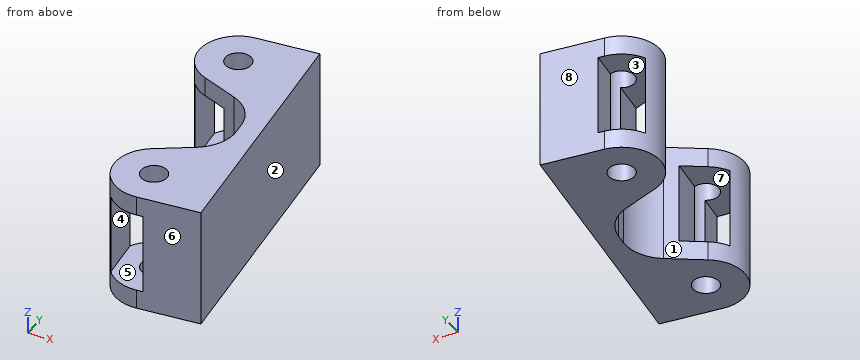
from build123d import *

# Parameters (mm, degrees)
SKETCH2_R           = 4
BOSS_EXTRUDE1_DEPTH = 18.5
SKETCH3_W           = 11.7897503
SKETCH3_H           = 96.005071975
CUT_EXTRUDE1_DEPTH  = 12.5


with BuildPart() as part:
    # Sketch2 → Boss-Extrude1 (new body, symmetric)
    with BuildSketch(Plane(origin=(137.548518754, -674.152855032, 0), x_dir=(0.993680552, 0.112245088, 0), z_dir=(0, 0, -1))):
        with BuildLine():
            Line((9.525, -304.744352791), (28.575, -304.744352791))
            Line((28.575, -304.744352791), (28.575, -387.05564726))
            Line((28.575, -387.05564726), (9.525993953, -387.05564726))
            ThreePointArc((9.525993953, -387.05564726), (-2.161189853, -377.777730047), (4.223746974, -364.290603044))
            Line((4.223746974, -364.290603044), (15.13654472, -358.9155811))
            ThreePointArc((15.13654472, -358.9155811), (20.308242044, -354.231651246), (22.225, -347.522575972))
            Line((22.225, -347.522575972), (22.225, -344.276661697))
            ThreePointArc((22.225, -344.276661697), (20.30793231, -337.567088625), (15.135492786, -332.883138506))
            Line((15.135492786, -332.883138506), (4.223746974, -327.509886515))
            ThreePointArc((4.223746974, -327.509886515), (-2.162309457, -314.022809542), (9.525, -304.744352791))
        make_face()
        with Locations((9.525993953, -375.05564726)):
            Circle(SKETCH2_R, mode=Mode.SUBTRACT)
        with Locations((9.525, -316.744352791)):
            Circle(SKETCH2_R, mode=Mode.SUBTRACT)
    extrude(amount=BOSS_EXTRUDE1_DEPTH, both=True)

    # Sketch3 → Cut-Extrude1 (cut, symmetric)
    with BuildSketch(Plane(origin=(140.134572942, -673.053475883, 0), x_dir=(0.993680552, 0.112245088, 0), z_dir=(0, 0, -1))):
        with Locations((2.760437102, -344.382335899)):
            Rectangle(SKETCH3_W, SKETCH3_H)
    extrude(amount=CUT_EXTRUDE1_DEPTH, both=True, mode=Mode.SUBTRACT)


solid = part.part
Geometry check sheet. Reference: the model listing, model coordinates, mm. Face numbers are marked on the shaded views. A direction names the side the tool comes from. Give positions to 0.01 mm unless a question says otherwise; leave off trailing zeros. Write each loop counter-clockwise with the first axis right and the second up, starting at its lowest first coordinate (ties: lowest second). Pieces come first, ordered by that corner, then holes.
1) Thickness scan on line 1 (Z direction, x = 111, y = -348.5); line 2 (Y direction, x = 113.5, z = 15); line 3 (X direction, y = -299.5, z = -11). Record the ranges inside material, lowest first.
Values follow:
line 1: z = -18.5 to -12.5, 12.5 to 18.5
line 2: y = -370.19 to -361.78, -354.9 to -342.78, -316.31 to -287.35
line 3: x = 92.95 to 94.78, 108.81 to 123.98
2) Release check for a two-part mould opening along X. For the marked faces 5, 6, 7 and 8 record: released by +X, released by -X, zero draft, split by the parting line, or undercut.
Values follow:
face 5: undercut
face 6: released by +X
face 7: undercut
face 8: released by -X
3) Cross-section at A-A (z = -3). Record the boundary of the cut face in (x, y), plus the area to 3 significant figures.
Values follow:
outline: (94.26, -294.88) arc R12 ccw to (95.76, -308.16) - close; (100.81, -352.82) arc R12 ccw to (102.31, -366.1) - close; (105.38, -288.27) - (106.33, -296.66) arc R4 cw to (107.13, -303.73) - (108.33, -314.38) - (112.3, -315.81) arc R12.7 cw to (120.63, -326.33) - (120.99, -329.56) arc R12.7 cw to (115.22, -341.67) - (111.67, -343.95) - (112.87, -354.6) arc R4 cw to (113.67, -361.67) - (114.62, -370.06) - (131.74, -368.13) - (122.5, -286.34) - close
area: 1,190 mm2
4) Cross-section at D-D (x = 97.5). Record the boundary of the cut face in (y, z).
Values follow:
outline: (-309.83, -18.5) - (-290.96, -18.5) - (-290.96, -12.5) - (-309.83, -12.5) - close; (-309.83, 12.5) - (-290.96, 12.5) - (-290.96, 18.5) - (-309.83, 18.5) - close
5) Cross-section at C-C (y = -360). Record the boundary of the cut face in (x, z), plus the area to 3 significant figures.
Values follow:
outline: (99.58, -18.5) - (107.82, -18.5) - (107.82, -12.5) - (101.62, -12.5) - (101.62, 12.5) - (107.82, 12.5) - (107.82, 18.5) - (99.58, 18.5) - close; (115.1, -18.5) - (130.82, -18.5) - (130.82, 18.5) - (115.1, 18.5) - close
area: 732 mm2
6) Cross-section at B-B (x = 110.5). Record the boundary of the cut face in (y, z).
Values follow:
outline: (-370.3, -18.5) - (-362.22, -18.5) - (-362.22, -12.5) - (-370.3, -12.5) - close; (-370.3, 12.5) - (-362.22, 12.5) - (-362.22, 18.5) - (-370.3, 18.5) - close; (-354.46, -18.5) - (-344.7, -18.5) - (-344.7, -12.5) - (-354.46, -12.5) - close; (-354.46, 12.5) - (-344.7, 12.5) - (-344.7, 18.5) - (-354.46, 18.5) - close; (-315.16, -18.5) - (-287.69, -18.5) - (-287.69, 18.5) - (-315.16, 18.5) - close
7) Go/stop test with flat-tipped pins: pin 1 Ø6 at (y, z) = (-325.5, -3.5) entering from -X; pin 2 Ø3 at (y, z) = (-350, 10) entering from -X; pin 3 Ø6 at (y, z) = (-335, -1) entering from -X. Record where each tip stops, or that it passes through.
Values follow:
pin 1: stops at x = 119.57
pin 2: stops at x = 112.18
pin 3: stops at x = 118.96
8) Set-up check for the marked faces 1, 2, 3 and 4: record each of +Z, -Z, +X, -X, +Y, -Y from which the full face is reachable in a straight line by a thin tool's end or side.
Values follow:
face 1: +Z, -Z, -X
face 2: +Z, -Z, +X, +Y
face 3: none
face 4: +Y
